Can you work these out from the drawing? Everything is in mm from the part's minimum corner. A direction names the side the tool comes from. Give positions to 0.01 mm unless a question says otherwise; leave off trailing zeros. Order: outer loops, then holes, each group sorted by start corner. A loop starts at its lowest first (then second) coordinate and runs counter-clockwise, first axis right, second up. Notation, with made-up numbers: (79.5, -35) - (107.5, -35) arc R31 cw to (107.5, -3) - close; hole circle Ø3 at (77, 34). An arc over 180 degrees is marked (long way). Answer as a JSON object with one key per item and string values.
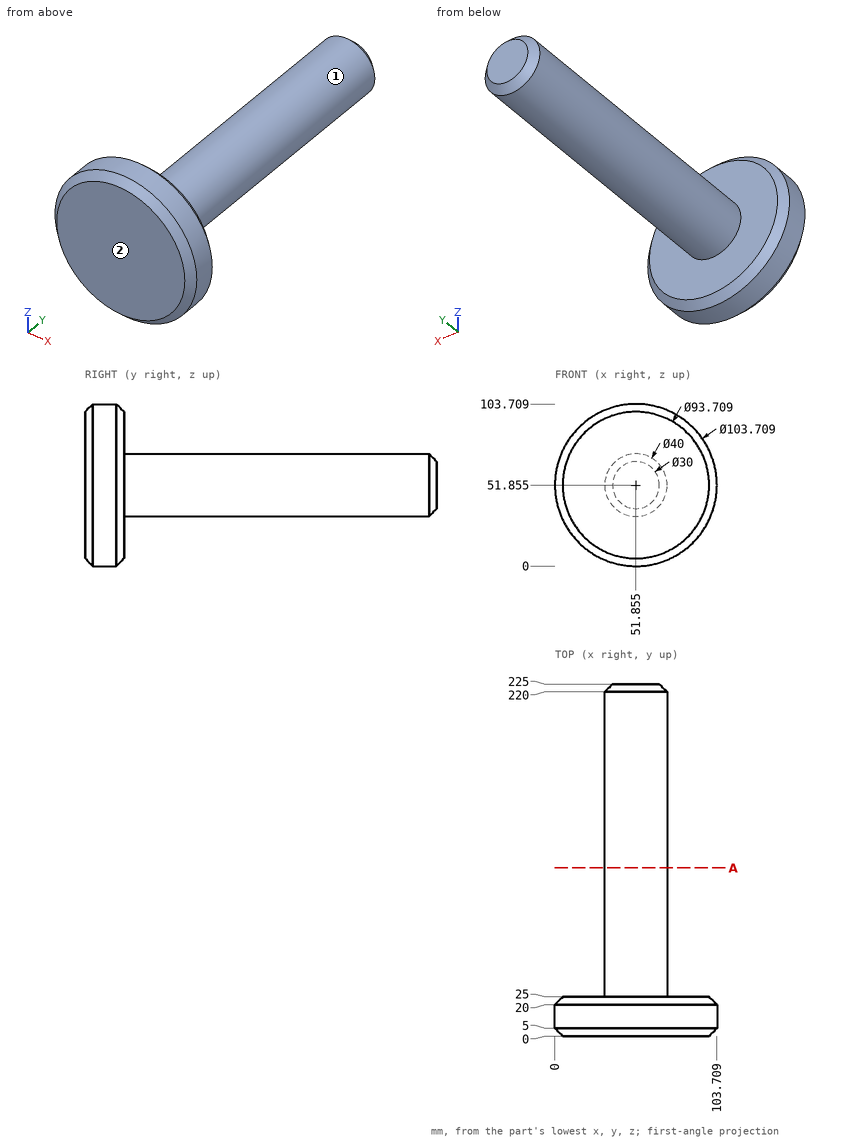
Q1. If we section it at A-A, the plane y = 107.5: Please give me the cut outline in (x, z) (1 decimal).
Recorded:
{"outline": "circle Ø40 at (51.9, 51.9)"}
Q2. Which directions (+Z, -Z, +X, -X, +Y, -Y) give clear straight access to the entire face, cutting with the end or side of a thin tool? Please do the marked faces 1 and 2.
Recorded:
{"face 1": "+Y", "face 2": "+Z, -Z, +X, -X, -Y"}
Q3. I'm going to push flat-ended pins straight in: pin 1 Ø10 at (x, z) = (64, 21) entering from +Y; pin 2 Ø6 at (y, z) = (144, 70.5) entering from +X (1 decimal); pin 3 Ø6 at (y, z) = (105, 58.5) entering from -X. Where does each tip first touch, or does it pass through?
Recorded:
{"pin 1": "stops at y = 25", "pin 2": "stops at x = 64.3", "pin 3": "stops at x = 32.19"}
Q4. I need wall thicknesses on L1, parallel to Y at x = 95, z = 52.5; L2, parallel to Y at x = 48, z = 35.5 (1 decimal); L3, parallel to Z at x = 58.5, y = 154.5. Which ranges of each line are inside material? Lowest first, please.
Recorded:
{"L1": "y = 0 to 25", "L2": "y = 0 to 223.2", "L3": "z = 32.99 to 70.72"}
